Geometry: see drawing. Coordinates: mm, zero at the bounding-box minimum. A direction names the side the tool comes from. Coordinates: 2 decimals unless noted, no trailing zeros. Write each loop counter-clockwise with the first axis right and the second up, starting at its lowest first coordinate (ties: lowest second). Pieces come first, ordered by that corner, then holes. Notation, with made-up numbers: (-21, 76.5) - (8, 76.5) arc R8 cw to (8, 83.5) - close; hole circle Ø11 at (-37.75, 65). An arc over 180 degrees is marked (long way). One line per question, with ' | ' between items. Start each with the question number.
1) Section query D-D on y = 57.15. Return loops of the section in (x, z) (1 decimal).
2) First-contact query: P1, Ø5, axis at x = 12.7, y = 57.15, coming from the +Z side (3 decimals); P2, Ø4, axis at y = 28, z = 53, coming from the +X side (3 decimals). Flat tips, straight axial feed; report the tip coordinate or a pass-through.
3) Reachability of the marked faces 1 and 2 from +Z, -Z, +X, -X, +Y, -Y: full face, straight path, thin tool, end or side. Return the list, or none.
4) Line query: line 1 (Y direction, x = 12.7, z = 1.4); line 2 (Z direction, x = 1.05, y = 44.45) (3 decimals); line 3 (Z direction, x = 3.5, y = 23) (3 decimals). Output: solid intervals per line, ascending.
5) Section query A-A on y = 82.55. Return loops of the section in (x, z) (1 decimal).
6) Section query C-C on x = 13. Return loops of the section in (y, z) (3 decimals).
7) Section query B-B on z = 38.1. Return loops of the section in (x, y) (3 decimals).
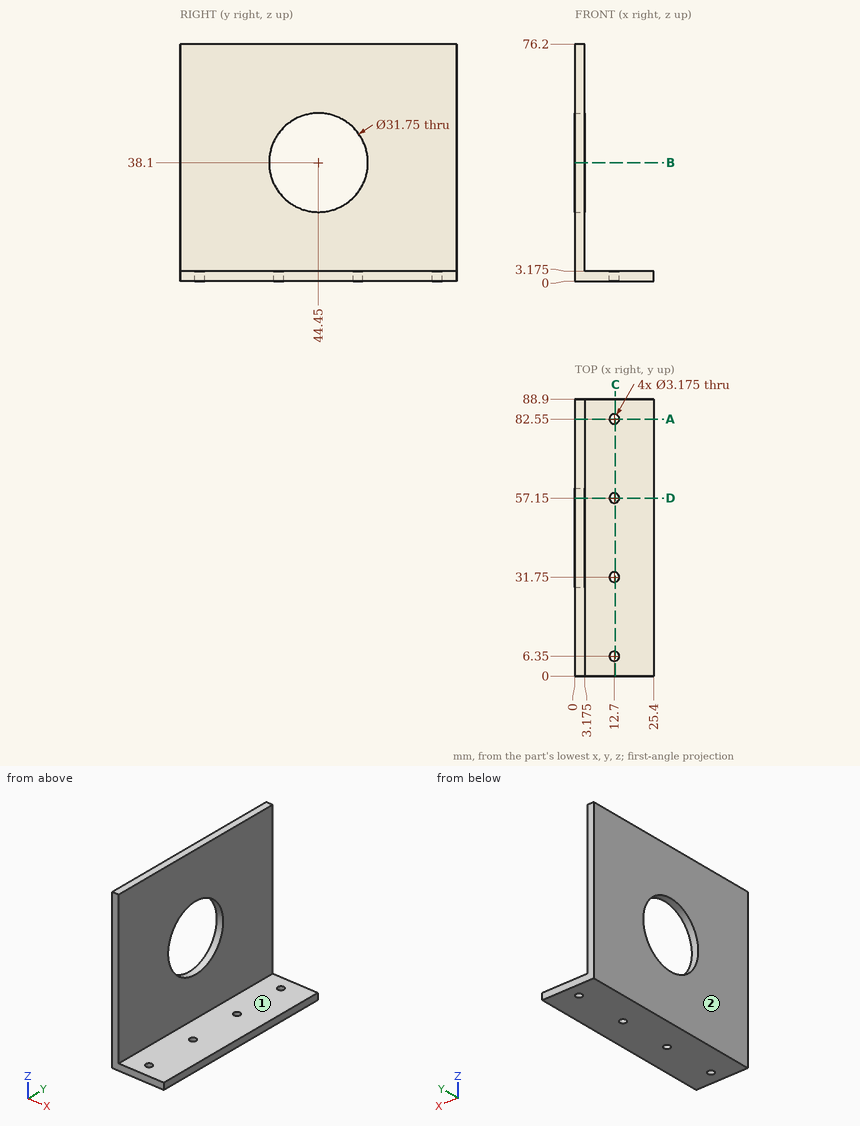
Answer key:
1) outline: (0, 0) - (11.1, 0) - (11.1, 3.2) - (3.2, 3.2) - (3.2, 28.6) - (0, 28.6) - close; (0, 47.6) - (3.2, 47.6) - (3.2, 76.2) - (0, 76.2) - close; (14.3, 0) - (25.4, 0) - (25.4, 3.2) - (14.3, 3.2) - close
2) P1: z = 3.175 | P2: x = 3.175
3) face 1: +Z, +X, +Y, -Y | face 2: +Z, -Z, -X, +Y, -Y
4) line 1: 0 to 4.76, 7.94 to 30.16, 33.34 to 55.56, 58.74 to 80.96, 84.14 to 88.9 | line 2: 0 to 22.225, 53.975 to 76.2 | line 3: 0 to 3.175
5) outline: (0, 0) - (11.1, 0) - (11.1, 3.2) - (3.2, 3.2) - (3.2, 76.2) - (0, 76.2) - close; (14.3, 0) - (25.4, 0) - (25.4, 3.2) - (14.3, 3.2) - close
6) outline: (0, 0) - (4.791, 0) - (4.791, 3.175) - (0, 3.175) - close; (7.909, 0) - (30.191, 0) - (30.191, 3.175) - (7.909, 3.175) - close; (33.309, 0) - (55.591, 0) - (55.591, 3.175) - (33.309, 3.175) - close; (58.709, 0) - (80.991, 0) - (80.991, 3.175) - (58.709, 3.175) - close; (84.109, 0) - (88.9, 0) - (88.9, 3.175) - (84.109, 3.175) - close
7) outline: (0, 0) - (3.175, 0) - (3.175, 28.575) - (0, 28.575) - close; (0, 60.325) - (3.175, 60.325) - (3.175, 88.9) - (0, 88.9) - close
